Part model, mm, in its own coordinate system. Round coordinates to 2 decimals unless told otherwise and drop trailing zeros. Loops run counter-clockwise (first coordinate to the right, second up) from the corner with the lowest first, then second, coordinate; pieces in that order, holes last.
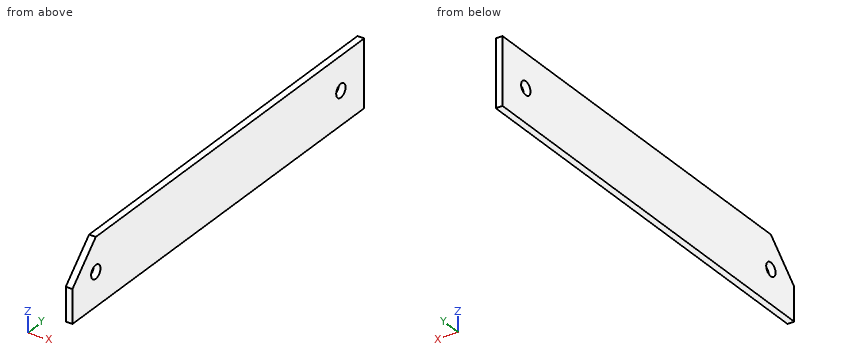
from build123d import *

# Parameters (mm, degrees)
SKETCH1_W           = 40
SKETCH1_H           = 250
SKETCH1_R           = 4
BOSS_EXTRUDE1_DEPTH = 4
CHAMFER3_SIZE       = 20


with BuildPart() as part:
    # Sketch1 → Boss-Extrude1 (new body)
    with BuildSketch(Plane(origin=(0, 0, 0), x_dir=(0, 0, -1), z_dir=(1, 0, 0))):
        Rectangle(SKETCH1_W, SKETCH1_H)
        with Locations((0, 105)):
            Circle(SKETCH1_R, mode=Mode.SUBTRACT)
        with Locations((0, -105)):
            Circle(SKETCH1_R, mode=Mode.SUBTRACT)
    extrude(amount=BOSS_EXTRUDE1_DEPTH)

    # Chamfer3
    chamfer3_edges = [part.edges().sort_by_distance(p)[0] for p in [
        (2, -125, 20),
    ]]
    chamfer(chamfer3_edges, length=CHAMFER3_SIZE)


solid = part.part
1) Wall check: line 1 along Y through (x, z) = (1.15, 0); line 2 along Y through (x, z) = (2.65, -2); line 3 along Z through (x, y) = (2.65, 106). Give the ranges that are in metal, low to high.
Values:
line 1: y = -125 to -109, -101 to 101, 109 to 125
line 2: y = -125 to -108.46, -101.54 to 101.54, 108.46 to 125
line 3: z = -20 to -3.87, 3.87 to 20
2) Slice it at B-B, the plane x = 1.75. Give the cut face in (y, z), then the cut area to 3 significant figures.
Values:
outline: (-125, -20) - (125, -20) - (125, 20) - (-105, 20) - (-125, 0) - close; hole circle Ø8 at (-105, 0); hole circle Ø8 at (105, 0)
area: 9,700 mm2
3) Slice it at A-A, the plane y = 105. Give the cut face in (x, z), then the cut area to 3 significant figures.
Values:
outline: (0, -20) - (4, -20) - (4, -4) - (0, -4) - close; (0, 4) - (4, 4) - (4, 20) - (0, 20) - close
area: 128 mm2
4) Slice it at C-C, the plane z = 10.5. Give the cut face in (x, y).
Values:
outline: (0, -114.5) - (4, -114.5) - (4, 125) - (0, 125) - close
